The model under review builds one solid part; all positions refer to its coordinate system, in mm. Round coordinates to 2 decimals unless told otherwise and drop trailing zeros. Write each loop counter-clockwise with the first axis right and the second up, starting at its lowest first coordinate (ties: lowest second). Pieces come first, ordered by that corner, then holes. Notation, with made-up numbers: (43.25, 58.5) - (102.25, 58.5) arc R21 cw to (102.25, 92.5) - close; hole circle Ø10 at (21.5, -12). An arc over 180 degrees is marked (long way). Return JSON: item names as keys, results as strings.
from build123d import *

# Parameters (mm, degrees)
CYLINDER001_R     = 8.4
CYLINDER001_DEPTH = 5.5
CYLINDER004_R     = 7.2
CYLINDER004_DEPTH = 6.5
CYLINDER003_R     = 10.4
CYLINDER003_DEPTH = 1
CYLINDER002_R     = 10.4
CYLINDER002_DEPTH = 2.75
SKETCH_R          = 8.4
SKETCH_R_2        = 1.8
SKETCH_R_3        = 3
PAD012_DEPTH      = 3.75


with BuildPart() as bearing_holder_extract:
    # Cylinder001 → Cylinder001 (new body)
    with BuildSketch(Plane.XY):
        Circle(CYLINDER001_R)
    extrude(amount=CYLINDER001_DEPTH)


with BuildPart() as bearing_holder_extract_fusion:
    # Cylinder004 → Cylinder004 (new body)
    with BuildSketch(Plane.XY.offset(-1)):
        Circle(CYLINDER004_R)
    extrude(amount=CYLINDER004_DEPTH)

    # Fusion001: union bearing holder extract
    add(bearing_holder_extract.part)


with BuildPart() as bearing_holder_disk:
    # Cylinder003 → Cylinder003 (new body)
    with BuildSketch(Plane.XY.offset(-1)):
        Circle(CYLINDER003_R)
    extrude(amount=CYLINDER003_DEPTH)


with BuildPart() as bearing_holder_body:
    # Cylinder002 → Cylinder002 (new body)
    with BuildSketch(Plane.XY):
        Circle(CYLINDER002_R)
    extrude(amount=CYLINDER002_DEPTH)

    # Fusion002: union bearing holder disk
    add(bearing_holder_disk.part)

    # Cut003: cut bearing holder extract fusion
    add(bearing_holder_extract_fusion.part, mode=Mode.SUBTRACT)


with BuildPart() as bearing_holder_body_1:
    # Cut003 placement: moved
    add(bearing_holder_body.part.moved(Location((0, 0, 1))))


with BuildPart() as bearing_holder_body_clone003:
    # Body012 base: copy of bearing holder body
    add(bearing_holder_body_1.part)


with BuildPart() as bearing_holder_body_clone003_1:
    # Body012 placement: moved
    add(bearing_holder_body_clone003.part.moved(Location((0, 25, 0))))


with BuildPart() as base_bearing_body:
    # Sketch → Pad012 (new body)
    with BuildSketch(Plane.XY):
        with BuildLine():
            Line((-44.05596, -13.84625), (-8.05596, 31.15375))
            ThreePointArc((8.186111, 31.15375), (0.065075, 35.056922), (-8.05596, 31.15375))
            Line((8.186111, 31.15375), (44.186111, -13.84625))
            ThreePointArc((36.065075, -30.743078), (45.438629, -24.848241), (44.186111, -13.84625))
            Line((36.065075, -30.743078), (-35.934925, -30.743078))
            ThreePointArc((-44.05596, -13.84625), (-45.308478, -24.848241), (-35.934925, -30.743078))
        make_face()
        with Locations((-35.934925, -20.343078)):
            Circle(SKETCH_R, mode=Mode.SUBTRACT)
        with Locations((0.065075, 24.656922)):
            Circle(SKETCH_R, mode=Mode.SUBTRACT)
        with Locations((36.065075, -20.343078)):
            Circle(SKETCH_R, mode=Mode.SUBTRACT)
        with Locations((-21.031229, 2.5)):
            Circle(SKETCH_R_2, mode=Mode.SUBTRACT)
        with Locations((20.961264, 2.5)):
            Circle(SKETCH_R_2, mode=Mode.SUBTRACT)
        with Locations((0, -22)):
            Circle(SKETCH_R_2, mode=Mode.SUBTRACT)
        with Locations((-27, 0.5)):
            Circle(SKETCH_R_3, mode=Mode.SUBTRACT)
    extrude(amount=PAD012_DEPTH)


with BuildPart() as base_bearing_fusion:
    # Body013 base: copy of bearing holder body
    add(bearing_holder_body_1.part)


with BuildPart() as base_bearing_fusion_1:
    # Body013 placement: moved
    add(base_bearing_fusion.part.moved(Location((36, -20, 0))))

    # Fusion004: union bearing holder body clone003, base bearing body
    add(bearing_holder_body_clone003_1.part)
    add(base_bearing_body.part)


with BuildPart() as part_mirroring:
    # Part__Mirroring: instance of base bearing fusion
    add(base_bearing_fusion_1.part.mirror(Plane(origin=(0, 0, 0), x_dir=(0, 1, 0), z_dir=(0, 0, 1))))


with BuildPart() as part_mirroring_1:
    # Part__Mirroring placement: moved
    add(part_mirroring.part.moved(Location((0, 0, 8))))


solid = part_mirroring_1.part
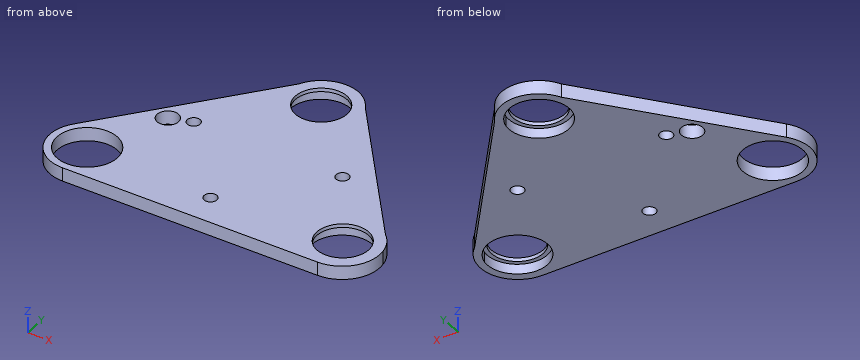
(1) Add section C-C (z = 5.1). Write out the cut boundary in (x, y), plus the area to 3 significant figures.
Filled in:
{"outline": "(-44.06, -13.85) arc R10.4 ccw to (-35.93, -30.74) - (36.07, -30.74) arc R10.4 ccw to (46.25, -18.23) arc R10.4 ccw to (42.85, -12.17) - (9.14, 29.96) arc R10.4 ccw to (-9.37, 29.51) - close; hole circle Ø16.8 at (-35.93, -20.34); hole circle Ø6 at (-27, 0.5); hole circle Ø3.6 at (-21.03, 2.5); hole (-8.22, 23.26) arc R8.4 ccw to (8.28, 26.39) arc R8.4 ccw to start; hole circle Ø3.6 at (0, -22); hole circle Ø3.6 at (20.96, 2.5); hole (27.78, -21.74) arc R8.4 ccw to (44.28, -18.61) arc R8.4 ccw to start", "area": "3,200 mm2"}
(2) Add section B-B (x = 0). Write out the cut boundary in (y, z).
Filled in:
{"outline": "(-30.74, 4.25) - (-23.8, 4.25) - (-23.8, 8) - (-30.74, 8) - close; (-20.2, 4.25) - (16.6, 4.25) - (16.6, 7) - (17.8, 7) - (17.8, 8) - (-20.2, 8) - close; (32.2, 7) - (33.06, 7) - (33.06, 4.25) - (35.4, 4.25) - (35.4, 8) - (32.2, 8) - close"}
(3) Add section A-A (y = 27.5). Write out the cut boundary in (x, z).
Filled in:
{"outline": "(-10.98, 4.25) - (-7.84, 4.25) - (-7.84, 7) - (-6.75, 7) - (-6.75, 8) - (-10.98, 8) - close; (6.75, 7) - (7.97, 7) - (7.97, 4.25) - (11.11, 4.25) - (11.11, 8) - (6.75, 8) - close"}
(4) Add section D-D (y = 13). Write out the cut boundary in (x, z).
Filled in:
{"outline": "(-22.58, 4.25) - (22.71, 4.25) - (22.71, 8) - (-22.58, 8) - close"}
(5) Clearance check with flat-ended pins moving along their axes: pin 1 Ø2 at (x, y) = (0, -22) entering from +Z; pin 2 Ø2 at (y, z) = (27, 5.5) entering from +X. State where each tip first meets the part, or that it passes through.
Filled in:
{"pin 1": "passes through", "pin 2": "stops at x = 12.31"}
(6) Wall thickness on line 1 (Y direction, x = 1, z = 6.75); line 2 (Y direction, x = 40, z = 6.9); line 3 (Y direction, x = -24.5, z = 6.9): over which ranges is each line inside the solid? List them lowest first.
Filled in:
{"line 1": "y = -30.74 to -23.5, -20.5 to 16.66, 33 to 35.35", "line 2": "y = -29.97 to -27.39, -12.92 to -8.61", "line 3": "y = -30.74 to -1.16, 2.16 to 10.6"}
